Geometry check sheet. Reference: the model listing, model coordinates, mm. A direction names the side the tool comes from. Coordinates: 2 decimals unless noted, no trailing zeros. Write each loop counter-clockwise with the first axis right and the second up, starting at its lowest first coordinate (ties: lowest second). Pieces come first, ordered by that corner, then holes. Notation, with made-up numbers: (53, 1) -> (58, 1) arc R29 ccw to (58, 33) -> close; hole circle Ø2 at (-15.5, 50). An arc over 180 degrees is marked (long way). Use a Markdown table: item, result.
```python
from build123d import *

# Parameters (mm, degrees)
F0_W      = 18
F0_H      = 7
F0_R      = 1.6
F1_DEPTH  = 15
F2_W      = 31
F2_H      = 5
F3_DEPTH  = 20
F4_R      = 1.5
F5_DEPTH  = 25
F6_R      = 1.5
F7_DEPTH  = 4.5
F8_R      = 1
F9_SIZE   = 5
F10_R     = 1.5
F11_DEPTH = 25


with BuildPart() as f1:
    # F0 (on Front) → F1 (new body)
    with BuildSketch(Plane.XZ):
        with Locations((9, 3.5)):
            Rectangle(F0_W, F0_H)
        with Locations((3, 3)):
            Circle(F0_R, mode=Mode.SUBTRACT)
        with Locations((15, 3)):
            Circle(F0_R, mode=Mode.SUBTRACT)
        Polygon((-6.5, 7), (0, 7), (18, 7), (24.5, 7), (24.5, 12), (0, 12), (-6.5, 12), align=None)
    extrude(amount=F1_DEPTH)

    # F2 (on face) → F3 (join)
    with BuildSketch(Plane.XY.offset(12)):
        with Locations((9, -2.5)):
            Rectangle(F2_W, F2_H)
    extrude(amount=F3_DEPTH)

    # F4 (on face) → F5 (cut)
    with BuildSketch(Plane.XZ.offset(5)):
        with Locations((2.75, 18)):
            Circle(F4_R)
        with Locations((15.25, 18)):
            Circle(F4_R)
    extrude(amount=-F5_DEPTH, mode=Mode.SUBTRACT)

    # F6 (on face) → F7 (cut)
    with BuildSketch(Plane.XY.offset(12)):
        with Locations((21.75, -11.5)):
            Circle(F6_R)
    extrude(amount=-F7_DEPTH, mode=Mode.SUBTRACT)

    # F8
    f8_edges = [f1.edges().sort_by_distance(p)[0] for p in [
        (0, -7.5, 0),
        (18, -7.5, 0),
        (0, -7.5, 7),
        (18, -7.5, 7),
    ]]
    fillet(f8_edges, radius=F8_R)

    # F9
    f9_edges = [f1.edges().sort_by_distance(p)[0] for p in [
        (24.5, -2.5, 32),
        (-6.5, -2.5, 32),
    ]]
    chamfer(f9_edges, length=F9_SIZE)

    # F10 (on face) → F11 (cut)
    with BuildSketch(Plane.XZ.offset(5)):
        with Locations((9.5, 26)):
            Circle(F10_R)
    extrude(amount=-F11_DEPTH, mode=Mode.SUBTRACT)


solid = f1.part
```
Item 1: Section check B-B on y = -2.5. Record the boundary of the cut face in (x, z).
Answer block:
| item | result |
|---|---|
| outline | (-6.5, 7) -> (-1, 7) arc R1 cw to (0, 6) -> (0, 1) arc R1 ccw to (1, 0) -> (17, 0) arc R1 ccw to (18, 1) -> (18, 6) arc R1 cw to (19, 7) -> (24.5, 7) -> (24.5, 27) -> (19.5, 32) -> (-1.5, 32) -> (-6.5, 27) -> close; hole circle Ø3 at (2.75, 18); hole circle Ø3.2 at (3, 3); hole circle Ø3 at (9.5, 26); hole circle Ø3.2 at (15, 3); hole circle Ø3 at (15.25, 18) |
Item 2: Mould release check, pull along Z, two halves, no side actions. Record for faces 4 (the flat face through (24.5, -4, 15)), 5 (the flat face through (-4, -2.5, 29.5)), 6 (the flat face through (9, -7, 0)), 7 (the cylindrical face through (14.14, -2.54, 19.01)): +Z half, -Z half, draft (parallel to the pull), parting line (faces both ways), or undercut.
Answer block:
| item | result |
|---|---|
| face 4 | draft |
| face 5 | +Z half |
| face 6 | -Z half |
| face 7 | undercut |
Item 3: Thickness scan on L1, parallel to Z at x = 15.25, y = -1.35; L2, parallel to Y at x = 21.75, z = 9.95; L3, parallel to Z at x = 3, y = -9.5. Record the ranges inside material, lowest first. Write a range as [from, to].
Answer block:
| item | result |
|---|---|
| L1 | z = [0, 1.42], [4.58, 16.5], [19.5, 32] |
| L2 | y = [-15, -13], [-10, 0] |
| L3 | z = [0, 1.4], [4.6, 12] |
Item 4: Section check C-C on x = 15. Record the boundary of the cut face in (y, z).
Answer block:
| item | result |
|---|---|
| outline | (-15, 0) -> (0, 0) -> (0, 1.4) -> (-15, 1.4) -> close; (-15, 4.6) -> (0, 4.6) -> (0, 16.52) -> (-5, 16.52) -> (-5, 12) -> (-15, 12) -> close; (-5, 19.48) -> (0, 19.48) -> (0, 32) -> (-5, 32) -> close |
Item 5: Tool access check on faces 1 (the cylindrical face through (20.25, -11.43, 9.78)), 2 (the flat face through (22, -7, 7)), 3 (the flat face through (0, -7, 3)). Record the directions out of +Z, -Z, +X, -X, +Y, -Y that give a thin tool (end or side, any length) a straight path to the whole face; none if there is none.
Answer block:
| item | result |
|---|---|
| face 1 | +Z |
| face 2 | -Z, +X, +Y, -Y |
| face 3 | -Z, -X, +Y, -Y |
Item 6: Depth check by flat-ended pin: P1, Ø4, axis at x = 11, y = -10, coming from the +Z side; P2, Ø1.6, axis at x = 21.5, y = -6, coming from the -Z side; P3, Ø5.5, axis at y = -7, z = 3.5, coming from the +X side. Enter the tip coordinate at first touch or a pass-through.
Answer block:
| item | result |
|---|---|
| P1 | stops at z = 12 |
| P2 | stops at z = 7 |
| P3 | stops at x = 18.03 |
Item 7: Section check D-D on y = -7.5. Record the boundary of the cut face in (x, z), then the cut area to 3 significant figures.
Answer block:
| item | result |
|---|---|
| outline | (-6.5, 7) -> (-1, 7) arc R1 cw to (0, 6) -> (0, 1) arc R1 ccw to (1, 0) -> (17, 0) arc R1 ccw to (18, 1) -> (18, 6) arc R1 cw to (19, 7) -> (24.5, 7) -> (24.5, 12) -> (-6.5, 12) -> close; hole circle Ø3.2 at (3, 3); hole circle Ø3.2 at (15, 3) |
| area | 265 mm^2 |
Item 8: Section check A-A on z = 3. Record the boundary of the cut face in (x, y), then the cut area to 3 significant figures.
Answer block:
| item | result |
|---|---|
| outline | (0, -15) -> (1.4, -15) -> (1.4, 0) -> (0, 0) -> close; (4.6, -15) -> (13.4, -15) -> (13.4, 0) -> (4.6, 0) -> close; (16.6, -15) -> (18, -15) -> (18, 0) -> (16.6, 0) -> close |
| area | 174 mm^2 |
